Input: dimensioned drawing with shaded views. Units: mm. Origin: part minimum x, y, z. Round coordinates to 2 decimals unless told otherwise and drop trailing zeros. Order: outer loops, then holes, each group sorted by start corner. A loop starts at its lowest first (then second) coordinate and runs counter-clockwise, first axis right, second up. Notation, with made-up numbers: (53.5, -28) - (112.5, -28) arc R20 ccw to (112.5, 1) - close; hole circle Ø10 at (83, 42.5). An arc over 180 degrees is marked (long way). Return JSON: item names as keys, results as strings. Group by question number.
1) Section B-B, the plane z = 20.5. Return loops of the section in (x, y).
2) Section A-A, the plane z = 15. Return loops of the section in (x, y), plus the area to 3 significant figures.
3) Ray query, line 1 (Y direction, x = 0.95, z = 15); line 2 (Y direction, x = 1.3, z = 18.75); line 3 (Z direction, x = 1.5, y = 22). Return the intervals inside material, ascending. Write a range as from..to.
4) Section C-C, the plane y = 6.5. Return loops of the section in (x, z), plus the area to 3 significant figures.
5) Section D-D, the plane x = 1.45. Return loops of the section in (y, z).
6) Contact query for a flat-ended pin moving along its axis: P1, Ø2.5, axis at y = 63.5, z = 15, coming from the -X side. Output: stop coordinate, or through.
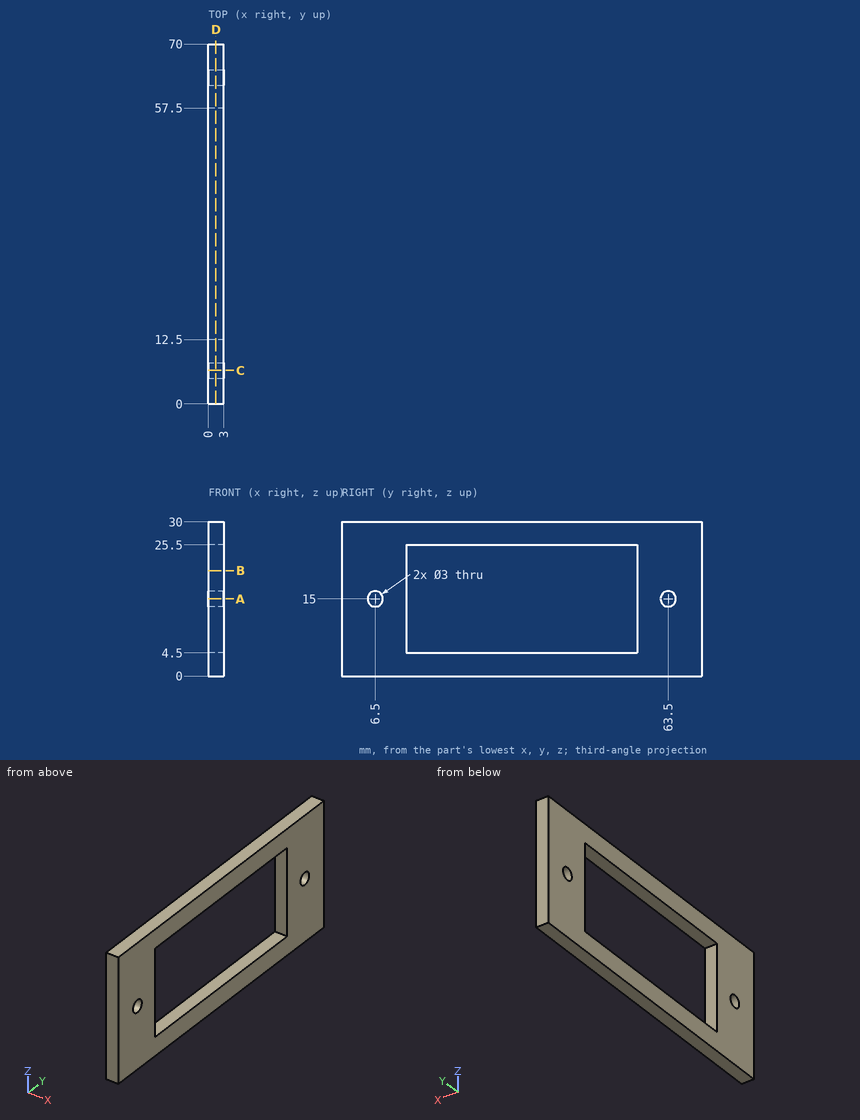
Geometry check:
{
 "1": {"outline": "(0, 0) - (3, 0) - (3, 12.5) - (0, 12.5) - close; (0, 57.5) - (3, 57.5) - (3, 70) - (0, 70) - close"},
 "2": {"outline": "(0, 0) - (3, 0) - (3, 5) - (0, 5) - close; (0, 8) - (3, 8) - (3, 12.5) - (0, 12.5) - close; (0, 57.5) - (3, 57.5) - (3, 62) - (0, 62) - close; (0, 65) - (3, 65) - (3, 70) - (0, 70) - close", "area": "57.0 mm2"},
 "3": {"line 1": "0..5, 8..12.5, 57.5..62, 65..70", "line 2": "0..12.5, 57.5..70", "line 3": "0..4.5, 25.5..30"},
 "4": {"outline": "(0, 0) - (3, 0) - (3, 13.5) - (0, 13.5) - close; (0, 16.5) - (3, 16.5) - (3, 30) - (0, 30) - close", "area": "81.0 mm2"},
 "5": {"outline": "(0, 0) - (70, 0) - (70, 30) - (0, 30) - close; hole circle Ø3 at (6.5, 15); hole (12.5, 4.5) - (57.5, 4.5) - (57.5, 25.5) - (12.5, 25.5) - close; hole circle Ø3 at (63.5, 15)"},
 "6": {"P1": "through"}
}
